Work out the finished part from the listing and answer in its coordinate system (mm). A direction names the side the tool comes from. Round coordinates to 2 decimals unless told otherwise and drop trailing zeros. Loops run counter-clockwise (first coordinate to the right, second up) from the corner with the lowest first, then second, coordinate; pieces in that order, holes last. Notation, with made-up numbers: (68.5, 40) - (98.5, 40) arc R20 ccw to (98.5, 66) - close; hole circle Ø6 at (12.5, -35). An arc over 180 degrees is marked (long way). Answer as CSV lines item,"result". Start each with the question number.
Q1. Section A-A on x = -11.25 is taken. Write down the section's boundary in (y, z), then the cut area to 3 significant figures.
Q2. Straight lines are drawn through the part: L1, parallel to Y at x = -14.75, z = 1.2; L2, parallel to Z at x = -2.25, y = 0; L3, parallel to Z at x = -7.75, y = -2.25. For each, find the intervals that lie inside material, in ascending order. Write a range as [from, to].
Q3. Section B-B on y = -0.25 is taken. Write down the section's boundary in (x, z), then the cut area to 3 significant figures.
Q4. Each of these flat-tipped pins is pushed along its axis until it touches: pin 1 Ø3 at (x, y) = (-4, -2) entering from +Z; pin 2 Ø1.5 at (x, y) = (-10.5, 4) entering from +Z; pin 3 Ø4 at (x, y) = (-3.5, 1.5) entering from -Z; pin 4 Ø0.6 at (y, z) = (1.5, 1) entering from -X. Where does it stop, or does it pass through?
Q5. For faces 4 (the face through (-3.94, 1.5, 0.81)), 5 (the face through (-8, -3.1, -1.2)), 6 (the face through (-9, 3, -2.65)), 7 (the face through (-3.94, 1.33, 2.39)), determine the directions among +Z, -Z, +X, -X, +Y, -Y from which every point of the face is accessible in a straight line to the end or side of a thin tool.
Q6. The mould has two halves that part along Y. Classify faces 1 (the face through (-9, 4, 2.65)), 2 (the face through (-9, 4, 2.15)), 3 (the face through (-9, 5.16, 0)): +Y half, -Y half, draft (parallel to the pull), parting line (faces both ways), or undercut.
Autodesk Inventor part; units mm, degrees
ref_plane "CP_XY" through (2, 5.16, 0) normal (1, 0, 0) x (0, 0, -1)
ref_plane "CP_YZ" through (2, 5.16, 0) normal (0, 0, -1) x (0, 1, 0)
ref_plane "CP_ZX" through (2, 5.16, 0) normal (0, 1, 0) x (1, 0, 0)
sketch "Sketch_11" plane through (0, 0, 0) normal (1, 0, 0) x (0, 1, 0)
  arc A0 (-1.1346, 2.5361) -> (-3.3951, 1.4765) centre (-1.84, 1.1) ccw
  arc A1 (-3.4923, 1.4) -> (-3.3951, 1.4765) centre (-3.4923, 1.5) ccw
  line L0 (-3.4923, 1.4) -> (-4.84, 1.4)
  arc A2 (-4.84, 1.4) -> (-5.14, 1.1) centre (-4.84, 1.1) ccw
  line L1 (-5.14, 1.1) -> (-5.14, -1.1)
  arc A3 (-5.14, -1.1) -> (-4.84, -1.4) centre (-4.84, -1.1) ccw
  line L2 (-4.84, -1.4) -> (-3.4923, -1.4)
  arc A4 (-3.3951, -1.4765) -> (-3.4923, -1.4) centre (-3.4923, -1.5) ccw
  arc A5 (-3.3951, -1.4765) -> (-1.1346, -2.5361) centre (-1.84, -1.1) ccw
  arc A6 (0.4796, -2.2735) -> (-1.1346, -2.5361) centre (0.1042, -5.0583) ccw
  line L3 (0.4796, -2.2735) -> (2.16, -2.5)
  line L4 (2.16, -2.5) -> (2.16, 2.5)
  line L5 (2.16, 2.5) -> (0.4796, 2.2735)
  arc A7 (-1.1346, 2.5361) -> (0.4796, 2.2735) centre (0.1042, 5.0583) ccw
  circle A8 centre (0, 0) radius 1.45
extrude "Extrusion1" add sketch "Sketch_11" against normal blind 8
sketch "Sketch_12" plane through (2, 0, 0) normal (1, 0, 0) x (0, 0, -1)
  line L0 (-2.65, 4.86) -> (-2.65, 2.16)
  line L1 (-2.65, 2.16) -> (2.65, 2.16)
  line L2 (2.65, 2.16) -> (2.65, 4.86)
  arc A0 (2.65, 4.86) -> (2.35, 5.16) centre (2.35, 4.86) ccw
  line L3 (2.35, 5.16) -> (-2.35, 5.16)
  arc A1 (-2.35, 5.16) -> (-2.65, 4.86) centre (-2.35, 4.86) ccw
extrude "Extrusion2" add sketch "Sketch_12" against normal blind 23
sketch "Sketch_13" plane through (2, 0, 0) normal (1, 0, 0) x (0, 0, -1)
  arc A0 (-2.15, 2.96) -> (-1.85, 2.66) centre (-1.85, 2.96) ccw
  line L0 (-1.85, 2.66) -> (1.85, 2.66)
  arc A1 (1.85, 2.66) -> (2.15, 2.96) centre (1.85, 2.96) ccw
  line L1 (2.15, 2.96) -> (2.15, 4.36)
  arc A2 (2.15, 4.36) -> (1.85, 4.66) centre (1.85, 4.36) ccw
  line L2 (1.85, 4.66) -> (-1.85, 4.66)
  arc A3 (-1.85, 4.66) -> (-2.15, 4.36) centre (-1.85, 4.36) ccw
  line L3 (-2.15, 4.36) -> (-2.15, 2.96)
extrude "Extrusion3" cut sketch "Sketch_13" against normal blind 23
sketch "Sketch_14" plane through (0, 0, 0) normal (1, 0, 0) x (0, 1, 0)
  arc A0 (-1.4233, 2.0091) -> (-2.84, 1.1) centre (-1.84, 1.1) ccw
  line L0 (-2.84, 1.1) -> (-2.84, 0.5446)
  arc A1 (-2.84, 0.5446) -> (-2.5075, 0.3948) centre (-2.64, 0.5446) ccw
  line L1 (-2.5075, 0.3948) -> (-1.3404, 1.4271)
  arc A2 (-1.0422, 1.09) -> (-1.3404, 1.4271) centre (-1.1913, 1.2585) ccw
  line L2 (-1.0422, 1.09) -> (-2.84, -0.5)
  line L3 (-2.84, -0.5) -> (-4.24, -0.5)
  arc A3 (-4.44, -0.3) -> (-4.24, -0.5) centre (-4.24, -0.3) ccw
  line L4 (-4.44, -0.3) -> (-4.44, 0.35)
  arc A4 (-4.24, 0.55) -> (-4.44, 0.35) centre (-4.24, 0.35) ccw
  arc A5 (-4.04, 0.35) -> (-4.24, 0.55) centre (-4.24, 0.35) ccw
  line L5 (-4.04, 0.35) -> (-4.04, 0.3)
  arc A6 (-4.04, 0.3) -> (-3.74, 0) centre (-3.74, 0.3) ccw
  arc A7 (-3.74, 0) -> (-3.44, 0.3) centre (-3.74, 0.3) ccw
  line L6 (-3.44, 0.3) -> (-3.44, 1.1)
  arc A8 (-3.1629, 2) -> (-3.44, 1.1) centre (-1.84, 1.1) ccw
  line L7 (-3.1629, 2) -> (-3.54, 2)
  line L8 (-3.54, 2) -> (-3.54, 0.3)
  arc A9 (-3.74, 0.1) -> (-3.54, 0.3) centre (-3.74, 0.3) ccw
  arc A10 (-3.94, 0.3) -> (-3.74, 0.1) centre (-3.74, 0.3) ccw
  line L9 (-3.94, 0.3) -> (-3.94, 0.4)
  arc A11 (-3.94, 0.4) -> (-4.14, 0.6) centre (-4.14, 0.4) ccw
  line L10 (-4.14, 0.6) -> (-4.34, 0.6)
  arc A12 (-4.34, 0.6) -> (-4.54, 0.4) centre (-4.34, 0.4) ccw
  line L11 (-4.54, 0.4) -> (-4.54, -0.6)
  arc A13 (-4.54, -0.6) -> (-4.34, -0.8) centre (-4.34, -0.6) ccw
  line L12 (-4.34, -0.8) -> (-3.4923, -0.8)
  arc A14 (-2.8119, -1.3353) -> (-3.4923, -0.8) centre (-3.4923, -1.5) ccw
  arc A15 (-2.8119, -1.3353) -> (-1.4233, -2.0091) centre (-1.84, -1.1) ccw
  arc A16 (-0.9842, -1.8433) -> (-1.4233, -2.0091) centre (-0.0025, -5.109) ccw
  line L13 (-0.9842, -1.8433) -> (-1.95, -0.6923)
  arc A17 (-1.6053, -0.403) -> (-1.95, -0.6923) centre (-1.7776, -0.5477) ccw
  line L14 (-1.6053, -0.403) -> (-0.4886, -1.7338)
  arc A18 (0.34, -1.7162) -> (-0.4886, -1.7338) centre (-0.0025, -5.109) ccw
  line L15 (0.34, -1.7162) -> (2.16, -1.9)
  line L16 (2.16, -1.9) -> (2.16, 1.9)
  line L17 (2.16, 1.9) -> (0.34, 1.7162)
  arc A19 (-1.4233, 2.0091) -> (0.34, 1.7162) centre (-0.0025, 5.109) ccw
extrude "Extrusion4" cut sketch "Sketch_14" against normal blind 8
sketch "Sketch_4" plane through (0, 0, 0) normal (1, 0, 0) x (0, 1, 0)
  line L0 (2.2363, -0.1854) -> (0.8628, -1.3489)
  line L1 (0.8628, -1.3489) -> (1.186, -1.7304)
  line L2 (1.186, -1.7304) -> (2.5595, -0.5669)
  line L3 (2.5595, -0.5669) -> (2.2363, -0.1854)
extrude "Extrusion5" add sketch "Sketch_4" against normal blind 8
sketch "Sketch_5" plane through (0, 0, 0) normal (1, 0, 0) x (0, 1, 0)
  line L0 (1.186, 1.7304) -> (0.8628, 1.3489)
  line L1 (0.8628, 1.3489) -> (2.2363, 0.1854)
  line L2 (2.2363, 0.1854) -> (2.5595, 0.5669)
  line L3 (2.5595, 0.5669) -> (1.186, 1.7304)
extrude "Extrusion6" add sketch "Sketch_5" against normal blind 8
ref_plane "CP_XY" through (2, 5.16, 0) normal (1, 0, 0) x (0, 0, -1)
ref_plane "CP_YZ" through (2, 5.16, 0) normal (0, 0, -1) x (0, 1, 0)
ref_plane "CP_ZX" through (2, 5.16, 0) normal (0, 1, 0) x (1, 0, 0)
ref_plane "KTN_XY" through (0, 0, 0) normal (1, 0, 0) x (0, 0, -1)
ref_plane "KTN_YZ" through (0, 0, 0) normal (0, 0, -1) x (0, 1, 0)
ref_plane "KTN_ZX" through (0, 0, 0) normal (0, 1, 0) x (1, 0, 0)
properties part number "1247168 ASCF-M-23-S DM 2.1-3.4"
Findings:
1,outline,"(2.16, -2.65) - (4.86, -2.65) arc R0.3 ccw to (5.16, -2.35) - (5.16, 2.35) arc R0.3 ccw to (4.86, 2.65) - (2.16, 2.65) - close; hole (2.66, -1.85) arc R0.3 ccw to (2.96, -2.15) - (4.36, -2.15) arc R0.3 ccw to (4.66, -1.85) - (4.66, 1.85) arc R0.3 ccw to (4.36, 2.15) - (2.96, 2.15) arc R0.3 ccw to (2.66, 1.85) - close"
1,area,"7.34 mm^2"
2,L1,"y = [2.16, 2.66], [4.66, 5.16]"
2,L2,"z = [-2.25, -1.7], [1.7, 2.25]"
2,L3,"z = [-2.65, -2.01], [0.02, 0.62], [2.01, 2.65]"
3,outline,"(-8, -2.27) - (0, -2.27) - (0, -1.71) - (-8, -1.71) - close; (-8, 1.71) - (0, 1.71) - (0, 2.27) - (-8, 2.27) - close"
3,area,"9.00 mm^2"
4,pin 1,"stops at z = 2.7"
4,pin 2,"stops at z = 2.65"
4,pin 3,"stops at z = -2.65"
4,pin 4,"stops at x = -8"
5,face 4,"+X, -X"
5,face 5,"+Z, -Z, -X, -Y"
5,face 6,"-Z, +X, -X, +Y"
5,face 7,"+Z, +X, -X"
6,face 1,"draft"
6,face 2,"undercut"
6,face 3,"+Y half"
